```python
from build123d import *

# Parameters (mm, degrees)
CBORE_FOR_M1_6_HEX_HEAD_CAP_SCREW1_D           = 3
CBORE_FOR_M1_6_HEX_HEAD_CAP_SCREW1_CBORE_D     = 5
CBORE_FOR_M1_6_HEX_HEAD_CAP_SCREW1_CBORE_DEPTH = 2
CIRPATTERN1_COUNT                              = 6
F_12_0MM_DOWEL_HOLE1_D                         = 12
F_12_0MM_DOWEL_HOLE1_DEPTH                     = 15
F_12_0MM_DOWEL_HOLE1_TIP                       = 3.605163714
CHAMFER1_SIZE                                  = 2
CIRPATTERN2_COUNT                              = 8


with BuildPart() as part:
    # Sketch1 → Revolve1 (revolve)
    with BuildSketch(Plane(origin=(0, 0, 0), x_dir=(0, 0, -1), z_dir=(1, 0, 0))):
        Polygon((0, 0), (0, 18.5), (12, 18.5), (12, 23.5), (11, 23.5), (11, 25.5), (12, 25.5), (12, 36.5), (9, 36.5), (9, 21.5), (-6, 21.5), (-6, 0), align=None)
    revolve(axis=Axis((0, 0, 6), (0, 0, -1)))

    # CBORE for M1.6 Hex Head Cap Screw1 (through all)
    with Locations(Plane.XY.offset(6)):
        with Locations((15.5, 0)):
            cbore_for_m1_6_hex_head_cap_screw1 = CounterBoreHole(CBORE_FOR_M1_6_HEX_HEAD_CAP_SCREW1_D / 2, CBORE_FOR_M1_6_HEX_HEAD_CAP_SCREW1_CBORE_D / 2, CBORE_FOR_M1_6_HEX_HEAD_CAP_SCREW1_CBORE_DEPTH)

    # CirPattern1: CBORE for M1.6 Hex Head Cap Screw1 ×6 about axis
    cirpattern1_axis = Axis((0, 0, 0), (0, 0, 1))
    for i in range(1, CIRPATTERN1_COUNT):
        add(cbore_for_m1_6_hex_head_cap_screw1.rotate(cirpattern1_axis, i * 360 / CIRPATTERN1_COUNT), mode=Mode.SUBTRACT)

    # Ø12.0mm Dowel Hole1
    with Locations(Plane.XY.offset(6)):
        with Locations((0, -7)):
            Hole(F_12_0MM_DOWEL_HOLE1_D / 2, depth=F_12_0MM_DOWEL_HOLE1_DEPTH)
            with Locations((0, 0, -(F_12_0MM_DOWEL_HOLE1_DEPTH + F_12_0MM_DOWEL_HOLE1_TIP / 2))):  # 118° drill point
                Cone(0, F_12_0MM_DOWEL_HOLE1_D / 2, F_12_0MM_DOWEL_HOLE1_TIP, mode=Mode.SUBTRACT)

    # Chamfer1
    chamfer1_edges = [part.edges().sort_by_distance(p)[0] for p in [
        (0, -21.5, 6),
        (0, -21.5, -9),
        (0, -36.5, -9),
    ]]
    chamfer(chamfer1_edges, length=CHAMFER1_SIZE)

    # Sketch7 → Ø3.0mm Dowel Hole3 (revolve, cut)
    with BuildSketch(Plane(origin=(0, 28, -9), x_dir=(0, -1, 0), z_dir=(1, 0, 0))):
        Polygon((0, 0), (0, 15.901290929), (1.5, 15), (1.5, 0), align=None)
    f_3_0mm_dowel_hole3 = revolve(axis=Axis((0, 28, -2.65), (0, 0, -1)), mode=Mode.SUBTRACT)

    # CirPattern2: Ø3.0mm Dowel Hole3 ×8 about axis
    cirpattern2_axis = Axis((0, 0, 0), (0, 0, 1))
    for i in range(1, CIRPATTERN2_COUNT):
        add(f_3_0mm_dowel_hole3.rotate(cirpattern2_axis, i * 360 / CIRPATTERN2_COUNT), mode=Mode.SUBTRACT)


solid = part.part
```
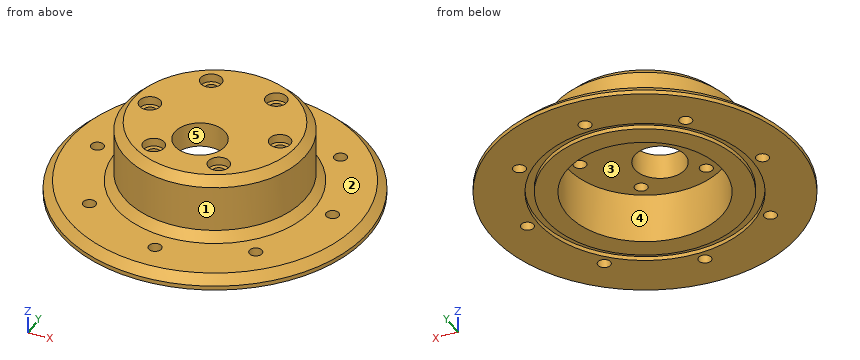
Model file for the job. Use its own axes, mm. Face numbers are marked on the shaded views. A direction names the side the tool comes from. Give positions to 0.01 mm unless a question says otherwise; leave off trailing zeros. Write each loop counter-clockwise with the first axis right and the second up, starting at its lowest first coordinate (ties: lowest second). Pieces come first, ordered by that corner, then holes. Notation, with made-up numbers: (11.5, 34.5) - (48.5, 34.5) arc R29 cw to (48.5, 61.5) - close; hole circle Ø10 at (42, 52). An arc over 180 degrees is marked (long way). One line per question, with ' | ' between items. Start each with the question number.
(1) Slice it at A-A on z = -2. Write the cut outline in (x, y), plus the area to 3 significant figures.
(2) Wall check: line 1 along Y through (x, z) = (7.75, 4.95); line 2 along Z through (x, y) = (-25.5, 21); line 3 along X through (y, z) = (12.5, -8.75). Give the ranges that are in metal, low to high. Write a range as from..to.
(3) Slice it at B-B on y = 0. Give the number of separate pieces and of enclosed holes in the cut face, plus the area to 3 significant figures.
(4) Pin check, flat tips, straight feed: P1, Ø5, axis at x = -15.5, y = 0, coming from the -Z side; P2, Ø8, axis at x = -21, z = -6, coming from the +Y side; P3, Ø8, axis at y = -5, z = -6, coming from the +X side. Stop position of each tip, or through.
(5) Two-plate mould, pull along Y, no slides. Class the marked faces 1, 2 and 3: +Y half, -Y half, draft (parallel to the pull), parting line (faces both ways), or undercut.
(6) 3-axis set-ups, long thin cutter, end or side, ignore diameter. For the marked faces 4 and 5: which of +Z, -Z, +X, -X, +Y, -Y reach the whole face in a straight line?
Results below:
1) outline: circle Ø43 at (0, 0); hole circle Ø37 at (0, 0) | area: 377 mm^2
2) line 1: -19.03..-15.92, -10.92..10.92, 15.92..19.03 | line 2: -12..-9 | line 3: -19.6..-13.64, 13.64..19.6
3) separate pieces: 5 | enclosed holes: 0 | area: 350 mm^2
4) P1: z = 0 | P2: y = 29.35 | P3: x = 35.18
5) face 1: parting line | face 2: draft | face 3: undercut
6) face 4: -Z | face 5: +Z, -Z
